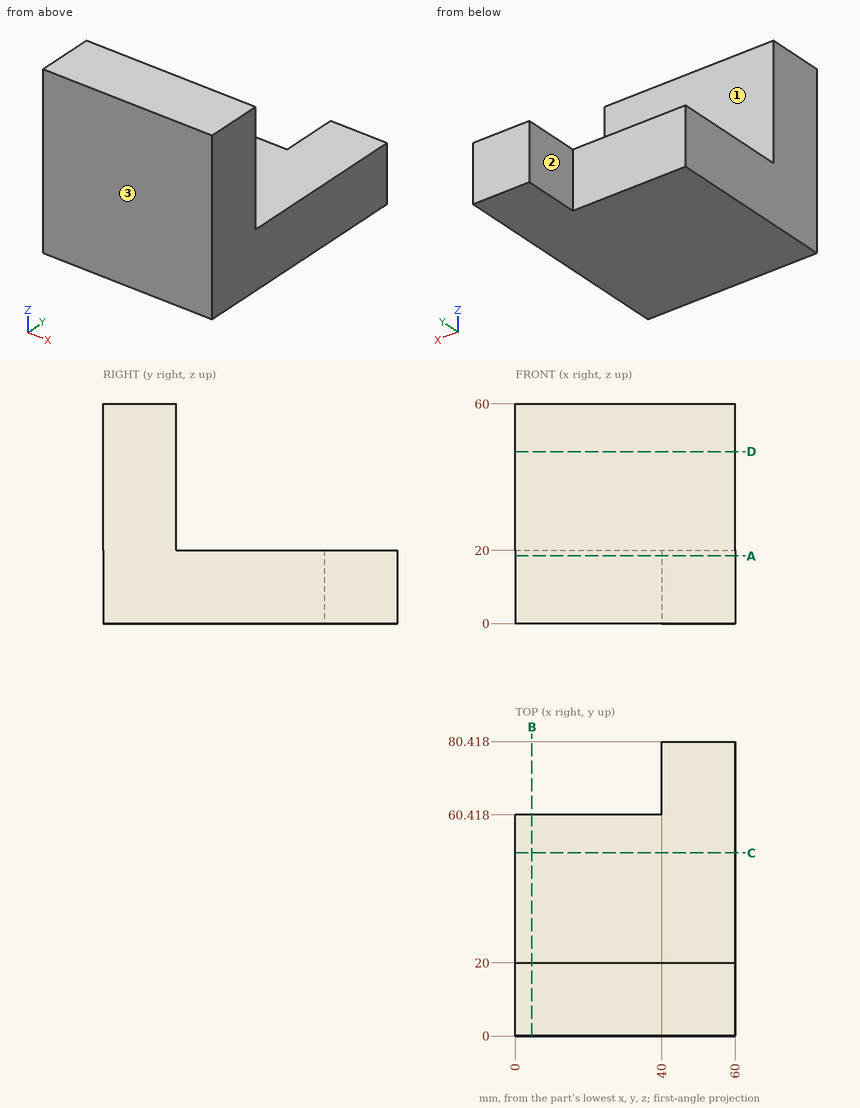
Print and shaded views of the part. All mm, measured from the part's lowest x, y and z. A direction names the side the tool comes from. Give positions to 0.01 mm unless a question says otherwise; leave off trailing zeros. Loops run counter-clockwise (first coordinate to the right, second up) from the corner with the lowest first, then second, coordinate; pieces in that order, holes last. Notation, with made-up numbers: (70, 79.5) - (114, 79.5) arc R21 cw to (114, 98.5) - close; hole circle Ø4 at (35.25, -2.75). An arc over 180 degrees is marked (long way). Use a Markdown table: item, result.
(1) Which spindle directions (+Z, -Z, +X, -X, +Y, -Y) get a long thin tool onto all of the face, cutting with end or side? Do the marked faces 1, 2 and 3. Say none if no direction does.
Taken from the geometry:
| item | result |
|---|---|
| face 1 | +Z, +X, -X, +Y |
| face 2 | +Z, -Z, -X, +Y |
| face 3 | +Z, -Z, +X, -X, -Y |
(2) Drop flat-ended pins along their axis: pin 1 Ø12 at (x, y) = (16.5, 67) entering from -Z; pin 2 Ø20 at (x, z) = (25, 41.5) entering from +Y; pin 3 Ø10 at (x, z) = (15.5, 14) entering from +Y; pin 4 Ø16 at (y, z) = (67.5, 13.5) entering from -X. Give the stop position or say it passes through.
Taken from the geometry:
| item | result |
|---|---|
| pin 1 | through |
| pin 2 | y = 20 |
| pin 3 | y = 60.42 |
| pin 4 | x = 0 |
(3) Band-saw the part on B-B (x = 4.5). Give the cut face in (y, z).
Taken from the geometry:
| item | result |
|---|---|
| outline | (0, 0) - (60.42, 0) - (60.42, 20) - (20, 20) - (20, 60) - (0, 60) - close |
(4) Band-saw the part on C-C (y = 50). Give the cut face in (x, z), and give its area (3 significant figures).
Taken from the geometry:
| item | result |
|---|---|
| outline | (0, 0) - (60, 0) - (60, 20) - (0, 20) - close |
| area | 1,200 mm2 |
(5) Band-saw the part on A-A (z = 18.5). Give the cut face in (x, y).
Taken from the geometry:
| item | result |
|---|---|
| outline | (0, 0) - (60, 0) - (60, 80.42) - (40, 80.42) - (40, 60.42) - (0, 60.42) - close |
(6) Wall check: line 1 along Y through (x, z) = (28, 45); line 2 along Y through (x, z) = (6, 11.5). Give the ranges that are in metal, low to high.
Taken from the geometry:
| item | result |
|---|---|
| line 1 | 0 to 20 |
| line 2 | 0 to 60.42 |
